Part print with two shaded views. Sizes in mm from the minimum x, y, z corner. A direction names the side the tool comes from. Give positions to 0.01 mm unless a question says otherwise; leave off trailing zeros. Write each loop counter-clockwise with the first axis right and the second up, starting at its lowest first coordinate (ties: lowest second). Pieces come first, ordered by that corner, then holes.
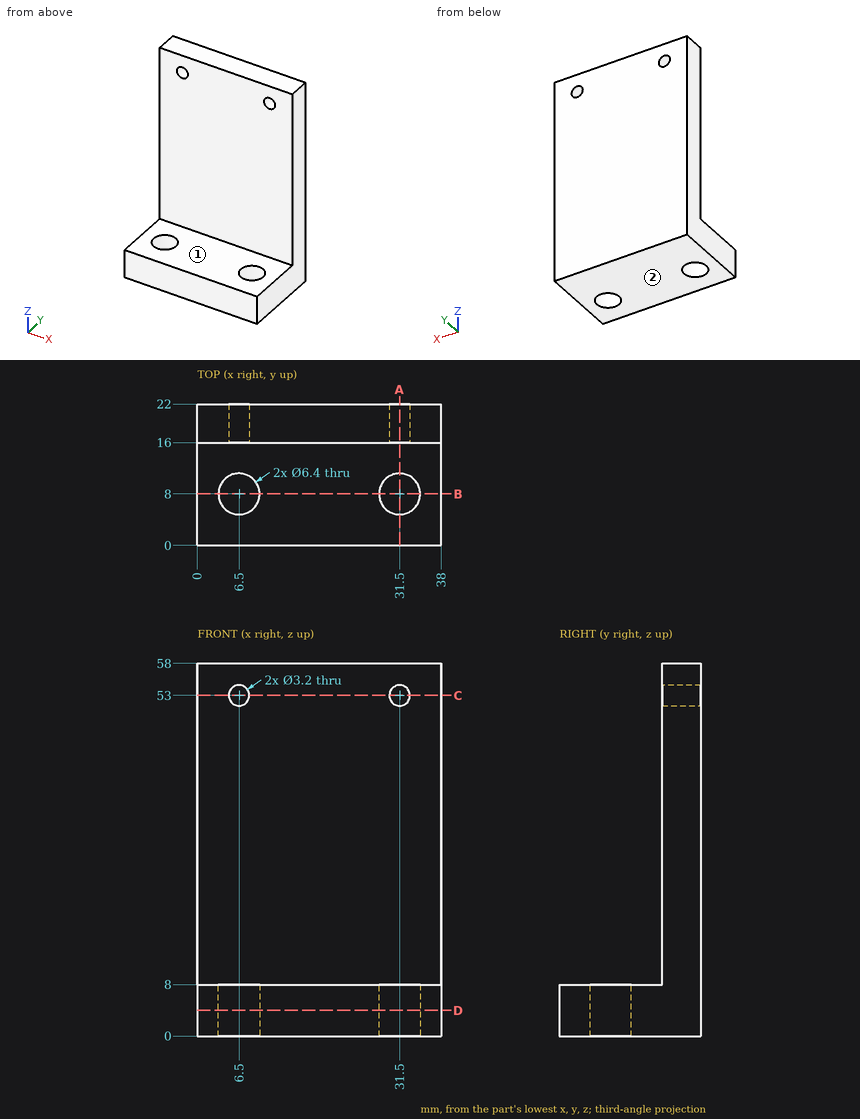
1) Saw through at B-B (y = 8). Write the cut outline in (x, z), and give its area (3 significant figures).
Check result:
outline: (0, 0) - (3.3, 0) - (3.3, 8) - (0, 8) - close; (9.7, 0) - (28.3, 0) - (28.3, 8) - (9.7, 8) - close; (34.7, 0) - (38, 0) - (38, 8) - (34.7, 8) - close
area: 202 mm2
2) Flat gauge pins, fed straight in: P1, Ø3, axis at x = 16.5, z = 12, coming from the -Y side; P2, Ø8.5, axis at x = 31.5, y = 8, coming from the +Z side. Where does each tip first touch, or does it go through?
Check result:
P1: stops at y = 16
P2: stops at z = 8
3) 3-axis set-ups, long thin cutter, end or side, ignore diameter. For the marked faces 1 and 2: which of +Z, -Z, +X, -X, +Y, -Y reach the whole face in a straight line?
Check result:
face 1: +Z, +X, -X, -Y
face 2: -Z, +X, -X, +Y, -Y
4) Saw through at A-A (x = 31.5). Write the cut outline in (y, z), and give its area (3 significant figures).
Check result:
outline: (0, 0) - (4.8, 0) - (4.8, 8) - (0, 8) - close; (11.2, 0) - (22, 0) - (22, 51.4) - (16, 51.4) - (16, 8) - (11.2, 8) - close; (16, 54.6) - (22, 54.6) - (22, 58) - (16, 58) - close
area: 406 mm2
5) Drill centre lines: L1, parallel to X at y = 18.5, z = 53; L2, parallel to Y at x = 11.5, z = 19; L3, parallel to X at y = 5.5, z = 6.5. Where is each one in solid material? Low to high.
Check result:
L1: x = 0 to 4.9, 8.1 to 29.9, 33.1 to 38
L2: y = 16 to 22
L3: x = 0 to 4.5, 8.5 to 29.5, 33.5 to 38
6) Saw through at D-D (z = 4). Write the cut outline in (x, y), and give its area (3 significant figures).
Check result:
outline: (0, 0) - (38, 0) - (38, 22) - (0, 22) - close; hole circle Ø6.4 at (6.5, 8); hole circle Ø6.4 at (31.5, 8)
area: 772 mm2
7) Saw through at C-C (z = 53). Write the cut outline in (x, y), and give its area (3 significant figures).
Check result:
outline: (0, 16) - (4.9, 16) - (4.9, 22) - (0, 22) - close; (8.1, 16) - (29.9, 16) - (29.9, 22) - (8.1, 22) - close; (33.1, 16) - (38, 16) - (38, 22) - (33.1, 22) - close
area: 190 mm2
